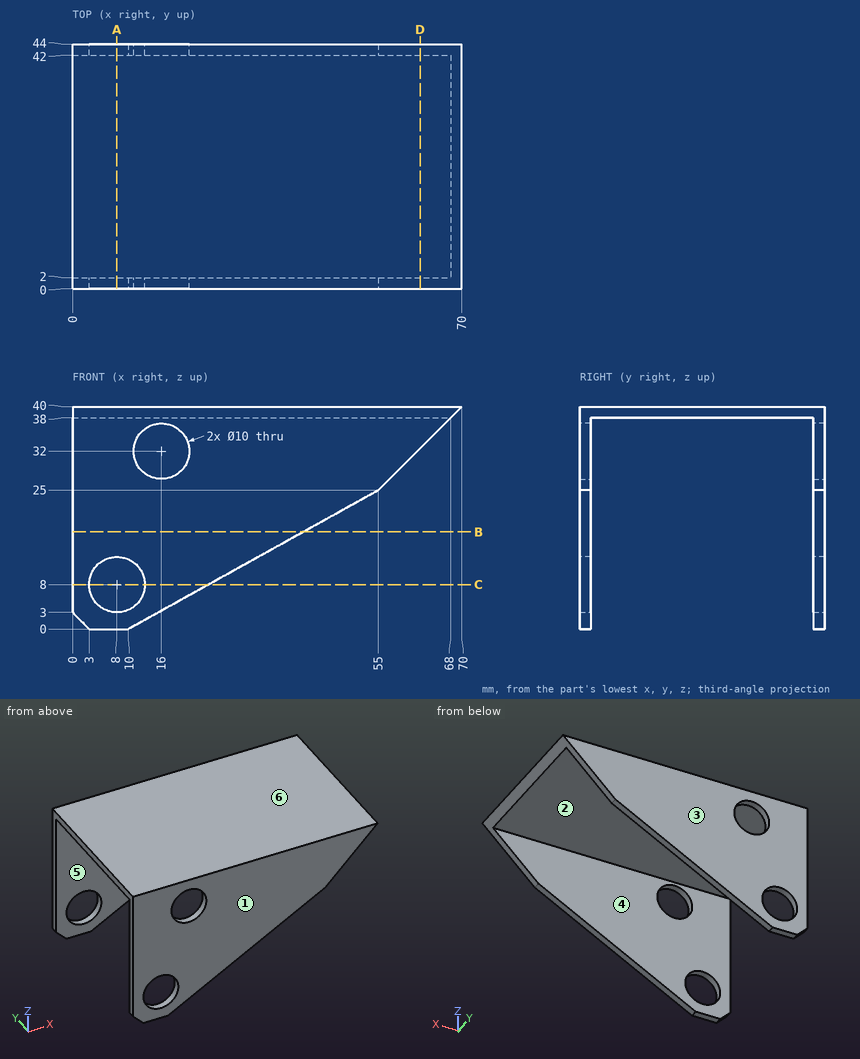
Could you check a few things on this drawing? It's one solid part, dimensions in mm from its lowest x, y, z. A direction names the side the tool comes from. Coordinates: 2 decimals unless noted, no trailing zeros. Order: outer loops, then holes, each group sorted by start corner. A loop starts at its lowest first (then second) coordinate and runs counter-clockwise, first axis right, second up. Notation, with made-up numbers: (77, 19) - (112, 19) arc R14 ccw to (112, 41) - close; hole circle Ø2 at (-31.5, -12.75). An arc over 180 degrees is marked (long way). Answer as a JSON object with one key per item and string values. Group by question number.
Q1. Will these pins go through, and if not, where does the flat tip stop? P1, Ø12, axis at x = 37.5, y = 7, coming from the -Z side; P2, Ø12, axis at x = 24.5, y = 28, coming from the -Z side; P3, Ø9, axis at x = 16, z = 32, coming from the -Y side (3 decimals).
Q2. Imagine slicing it at D-D (x = 62.5). Please give me the cut outline in (y, z).
Q3. I need wall thicknesses on line 1 (Y direction, x = 34, z = 15); line 2 (Z direction, x = 47, y = 22.5); line 3 (X direction, y = 43.05, z = 32). Which ranges of each line are inside material? Lowest first, please. Write a range as from..to.
Q4. Imagine slicing it at A-A (x = 8). Please give me the cut outline in (y, z).
Q5. We'd pull the mould along Y, two halves only. Please class the marked faces 3, 4, 5 and 6: +Y half, -Y half, draft (parallel to the pull), parting line (faces both ways), or undercut.
Q6. On a 3-axis mill with a long thin cutter (end or side, diameter ignored), from which of +Z, -Z, +X, -X, +Y, -Y can I reach the whole of each face in a straight line? I mean the marked faces 1 and 2. Say none if no direction works.
Q7. Imagine slicing it at C-C (z = 8). Please give me the cut outline in (x, y).
Q8. Imagine slicing it at B-B (z = 17.5). Please give me the cut outline in (x, y), and give its area (3 significant figures).
Determined:
{
 "1": {"P1": "stops at z = 13.44", "P2": "stops at z = 38", "P3": "passes through"},
 "2": {"outline": "(0, 32.5) - (2, 32.5) - (2, 38) - (42, 38) - (42, 32.5) - (44, 32.5) - (44, 40) - (0, 40) - close"},
 "3": {"line 1": "y = 0..2, 42..44", "line 2": "z = 38..40", "line 3": "x = 0..11, 21..62"},
 "4": {"outline": "(0, 0) - (2, 0) - (2, 3) - (0, 3) - close; (0, 13) - (2, 13) - (2, 38) - (42, 38) - (42, 13) - (44, 13) - (44, 40) - (0, 40) - close; (42, 0) - (44, 0) - (44, 3) - (42, 3) - close"},
 "5": {"face 3": "+Y half", "face 4": "undercut", "face 5": "undercut", "face 6": "draft"},
 "6": {"face 1": "+Z, -Z, +X, -X, -Y", "face 2": "-Z, +X, -X"},
 "7": {"outline": "(0, 0) - (3, 0) - (3, 2) - (0, 2) - close; (0, 42) - (3, 42) - (3, 44) - (0, 44) - close; (13, 0) - (24.4, 0) - (24.4, 2) - (13, 2) - close; (13, 42) - (24.4, 42) - (24.4, 44) - (13, 44) - close"},
 "8": {"outline": "(0, 0) - (41.5, 0) - (41.5, 2) - (0, 2) - close; (0, 42) - (41.5, 42) - (41.5, 44) - (0, 44) - close", "area": "166 mm2"}
}
